Geometry check sheet. Reference: the model listing, model coordinates, mm. A direction names the side the tool comes from. Coordinates: 2 decimals unless noted, no trailing zeros. Order: outer loops, then holes, each group sorted by start corner. A loop starts at its lowest first (then second) coordinate and runs counter-clockwise, first axis right, second up. Notation, with made-up numbers: (35.25, 52) - (91.25, 52) arc R18 cw to (91.25, 79) - close; hole circle Ø8 at (51, 7). An arc over 180 degrees is marked (long way). Return JSON: item names as keys, results as strings. Group by question number.
Item 1: Section check D-D on y = -5. Enter the section's corners in (x, z).
Item 2: Scan lines: probe 1 along X at (y, z) = (3.1, 6); probe 2 along X at (y, z) = (-8.5, 0); probe 3 along Y at (x, z) = (9.5, -8.25). Record each from-to range of solid material in increasing order.
Item 3: Tool access check on faces 4 (the flat face through (6, 1.577, -6)), 5 (the flat face through (5.2, -18.423, 0.1)). Record the directions out of +Z, -Z, +X, -X, +Y, -Y that give a thin tool (end or side, any length) a straight path to the whole face; none if there is none.
Item 4: Gauge pin test, flat ends, axial feed: pin 1 (4 mm diameter, centred on x = -7, z = 9, fed in from -Y); pin 2 (6 mm diameter, centred on x = 7, y = 1.5, fed in from +Z); pin 3 (8 mm diameter, centred on x = -11, y = -10.5, fed in from +Z); pin 4 (10 mm diameter, centred on x = -6.5, z = 8, fed in from -Y). Record the tip position at first contact, or that the pin passes through.
Item 5: Draft check along X on faces 1 (the flat face through (-4, 6.827, -4)), 2 (the cylindrical face through (4.88, -5.97, -1.08)), 3 (the cylindrical face through (7.81, -8.28, -1.73)). Enter one of: pulls with the +X half, pulls with the -X half, needs draft (parallel to the pull), parting line crosses it, or undercut.
Item 6: Section check A-A on x = 0. Enter the section's corners in (y, z), then the cut area to 3 significant figures.
Item 7: Section check B-B on z = 0. Enter the section's corners in (x, y).
Item 8: Section check C-C on x = -10.75. Enter the section's corners in (y, z).
from build123d import *

# Parameters (mm, degrees)
SKETCH2_R          = 1.5
CUT_EXTRUDE1_DEPTH = 10
CIRPATTERN1_COUNT  = 3


with BuildPart() as part:
    # Sketch1 → Revolve1 (revolve)
    with BuildSketch(Plane.XY, mode=Mode.PRIVATE) as revolve1_sk:
        Polygon((-5, 6.826923077), (-5, -18.423076923), (-8, -18.423076923), (-8, 1.576923077), (-15, 1.576923077), (-15, 6.826923077), align=None)
    revolve(revolve1_sk.sketch.rotate(Axis((0, 6, 0), (0, -1, 0)), 270), axis=Axis((0, 6, 0), (0, -1, 0)))

    # Sketch2 → Cut-Extrude1 (cut)
    with BuildSketch(Plane(origin=(0, 6.826923077, 0), x_dir=(1, 0, 0), z_dir=(0, 1, 0))):
        with Locations(Location((0, 12, 0), (0, 0, 270))):
            Circle(SKETCH2_R)
    cut_extrude1 = extrude(amount=-CUT_EXTRUDE1_DEPTH, mode=Mode.SUBTRACT)

    # CirPattern1: Cut-Extrude1 ×3 about axis
    cirpattern1_axis = Axis((0, 0, 0), (0, 1, 0))
    for i in range(1, CIRPATTERN1_COUNT):
        add(cut_extrude1.rotate(cirpattern1_axis, i * 360 / CIRPATTERN1_COUNT), mode=Mode.SUBTRACT)


solid = part.part
Computed:
{
 "1": {"outline": "circle Ø16 at (0, 0); hole circle Ø10 at (0, 0)"},
 "2": {"probe 1": "x = -13.75 to -11.89, -8.89 to 8.89, 11.89 to 13.75", "probe 2": "x = -8 to -5, 5 to 8", "probe 3": "y = 1.58 to 6.83"},
 "3": {"face 4": "-Y", "face 5": "+Z, -Z, +X, -X, -Y"},
 "4": {"pin 1": "stops at y = 1.58", "pin 2": "stops at z = 14.46", "pin 3": "stops at z = 3.87", "pin 4": "stops at y = -18.42"},
 "5": {"face 1": "needs draft", "face 2": "undercut", "face 3": "parting line crosses it"},
 "6": {"outline": "(-18.42, -8) - (1.58, -8) - (1.58, -10.5) - (6.83, -10.5) - (6.83, -5) - (-18.42, -5) - close; (-18.42, 5) - (6.83, 5) - (6.83, 15) - (1.58, 15) - (1.58, 8) - (-18.42, 8) - close; (1.58, -15) - (6.83, -15) - (6.83, -13.5) - (1.58, -13.5) - close", "area": "209 mm²"},
 "7": {"outline": "(-15, 1.58) - (-8, 1.58) - (-8, -18.42) - (-5, -18.42) - (-5, 6.83) - (-15, 6.83) - close; (5, -18.42) - (8, -18.42) - (8, 1.58) - (15, 1.58) - (15, 6.83) - (5, 6.83) - close"},
 "8": {"outline": "(1.58, -10.46) - (6.83, -10.46) - (6.83, 4.54) - (1.58, 4.54) - close; (1.58, 7.46) - (6.83, 7.46) - (6.83, 10.46) - (1.58, 10.46) - close"}
}
